from build123d import *

# Parameters (mm, degrees)
SKETCH1_W           = 10
SKETCH1_H           = 32
BOSS_EXTRUDE1_DEPTH = 6
SKETCH2_W           = 10
SKETCH2_H           = 20
BOSS_EXTRUDE2_DEPTH = 6
SKETCH3_R           = 2.25
CUT_EXTRUDE1_DEPTH  = 13
SKETCH4_R           = 4
CUT_EXTRUDE2_DEPTH  = 4
CHAMFER1_SIZE       = 3
CHAMFER2_SIZE       = 0.5
SKETCH5_R           = 2.727238267
CUT_EXTRUDE3_DEPTH  = 7


with BuildPart() as part:
    # Sketch1 → Boss-Extrude1 (new body)
    with BuildSketch(Plane.XY):
        with Locations((5, -16)):
            Rectangle(SKETCH1_W, SKETCH1_H)
    extrude(amount=BOSS_EXTRUDE1_DEPTH)

    # Sketch2 → Boss-Extrude2 (add)
    with BuildSketch(Plane.XY.offset(6)):
        with Locations((5, -10)):
            Rectangle(SKETCH2_W, SKETCH2_H)
    extrude(amount=BOSS_EXTRUDE2_DEPTH)

    # Sketch3 → Cut-Extrude1 (cut, through all)
    with BuildSketch(Plane.XY.offset(12)):
        with Locations((5, -4.5)):
            Circle(SKETCH3_R)
        with Locations((5, -14.5)):
            Circle(SKETCH3_R)
    extrude(amount=-CUT_EXTRUDE1_DEPTH, mode=Mode.SUBTRACT)

    # Sketch4 → Cut-Extrude2 (cut)
    with BuildSketch(Plane.XY.offset(12)):
        with Locations((5, -4.5)):
            Circle(SKETCH4_R)
        with Locations((5, -14.5)):
            Circle(SKETCH4_R)
    extrude(amount=-CUT_EXTRUDE2_DEPTH, mode=Mode.SUBTRACT)

    # Chamfer1
    chamfer1_edges = [part.edges().sort_by_distance(p)[0] for p in [
        (10, -32, 3),
        (0, -32, 3),
    ]]
    chamfer(chamfer1_edges, length=CHAMFER1_SIZE)

    # Chamfer2
    chamfer2_edges = [part.edges().sort_by_distance(p)[0] for p in [
        (0, -10, 12),
        (10, -10, 12),
    ]]
    chamfer(chamfer2_edges, length=CHAMFER2_SIZE)

    # Sketch5 → Cut-Extrude3 (cut, through all)
    with BuildSketch(Plane.XY.offset(6)):
        with Locations((5, -26)):
            Circle(SKETCH5_R)
    extrude(amount=-CUT_EXTRUDE3_DEPTH, mode=Mode.SUBTRACT)


solid = part.part
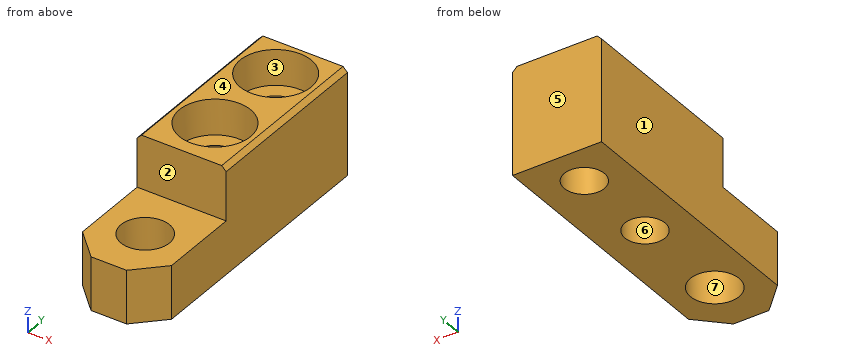
For this review, take the finished solid that the model builds, in its own axes (mm). Face numbers are marked on the shaded views. A direction names the side the tool comes from. Round coordinates to 2 decimals unless told otherwise and drop trailing zeros. Order: outer loops, then holes, each group sorted by start corner. A loop starts at its lowest first (then second) coordinate and runs counter-clockwise, first axis right, second up. Notation, with made-up numbers: M 3,23 L 23,23 A24 cw 23,43 Z; hole C 69,89 d2. An arc over 180 degrees is marked long. Use a Markdown table: item, result. Add a question column.
Item 1: Insertion check: pin 1 (5 mm diameter, centred on x = 5, y = -14.5, fed in from +Z); pin 2 (3 mm diameter, centred on x = 8.5, z = 9, fed in from -Y). Each pin has a flat end and moves straight along its axis. Give the tip position at first contact, or say it passes through.
Item 2: To check wall thickness, follow line 1 along Y through (x, z) = (5, 11.15); line 2 along Y through (x, z) = (5, 1.8); line 3 along X through (y, z) = (-2.5, 2.5). State the ranges of each line that lie inside material, in increasing order.
Item 3: Mouldability with a two-part tool opening along Y and no side actions: class the marked faces 4, 5, 6 and 7 as released by +Y, released by -Y, zero draft, split by the parting line, or undercut.
Item 4: Add section D-D, the plane z = 10.25. Give the boundary of the cut face in (x, y), then the cut area to 3 significant figures.
Item 5: Add section A-A, the plane z = 5.25. Give the boundary of the cut face in (x, y), then the cut area to 3 significant figures.
Item 6: Add section B-B, the plane x = 5. Give the boundary of the cut face in (y, z), then the cut area to 3 significant figures.
Item 7: Add section C-C, the plane y = -26. Give the boundary of the cut face in (x, z).
Item 8: Tool access review of the marked faces 1, 2 and 3: name each direction out of +Z, -Z, +X, -X, +Y, -Y from which nothing blocks a thin tool from reaching the whole face with its end or side.
Geometry results:
| question | item | result |
|---|---|---|
| 1 | pin 1 | stops at z = 8 |
| 1 | pin 2 | stops at y = -20 |
| 2 | line 1 | y = -20 to -18.5, -10.5 to -8.5, -0.5 to 0 |
| 2 | line 2 | y = -32 to -28.73, -23.27 to -16.75, -12.25 to -6.75, -2.25 to 0 |
| 2 | line 3 | x = 0 to 3.97, 6.03 to 10 |
| 3 | face 4 | zero draft |
| 3 | face 5 | released by +Y |
| 3 | face 6 | undercut |
| 3 | face 7 | undercut |
| 4 | outline | M 0,-20 L 10,-20 L 10,0 L 0,0 Z; hole C 5,-14.5 d8; hole C 5,-4.5 d8 |
| 4 | area | 99.5 mm² |
| 5 | outline | M 0,-29 L 3,-32 L 7,-32 L 10,-29 L 10,0 L 0,0 Z; hole C 5,-26 d5.45; hole C 5,-14.5 d4.5; hole C 5,-4.5 d4.5 |
| 5 | area | 256 mm² |
| 6 | outline | M -32,0 L -28.73,0 L -28.73,6 L -32,6 Z; M -23.27,0 L -16.75,0 L -16.75,8 L -18.5,8 L -18.5,12 L -20,12 L -20,6 L -23.27,6 Z; M -12.25,0 L -6.75,0 L -6.75,8 L -8.5,8 L -8.5,12 L -10.5,12 L -10.5,8 L -12.25,8 Z; M -2.25,0 L 0,0 L 0,12 L -0.5,12 L -0.5,8 L -2.25,8 Z |
| 6 | area | 143 mm² |
| 7 | outline | M 0,0 L 2.27,0 L 2.27,6 L 0,6 Z; M 7.73,0 L 10,0 L 10,6 L 7.73,6 Z |
| 8 | face 1 | +Z, -Z, -X, +Y, -Y |
| 8 | face 2 | +Z, +X, -X, -Y |
| 8 | face 3 | +Z |
